from build123d import *

# Parameters (mm, degrees)
CROQUIS1_R                 = 8
SALIENTE_EXTRUIR1_DEPTH    = 20
CORTAR_EXTRUIR1_DEPTH      = 8.5
CROQUIS3_R                 = 6.75
CORTAR_EXTRUIR2_DEPTH      = 9
CORTAR_EXTRUIR3_REACH      = 17.78
CROQUIS4_R                 = 2.025
CORTAR_EXTRUIR4_DEPTH      = 9
CORTAR_EXTRUIR4_DEPTH_BACK = 23.978250586
CROQUIS5_R                 = 2
SALIENTE_EXTRUIR2_START    = 7
CROQUIS6_R                 = 8
CROQUIS6_R_2               = 6.75
SALIENTE_EXTRUIR2_DEPTH    = 7


with BuildPart() as part:
    # Croquis1 → Saliente-Extruir1 (new body)
    with BuildSketch(Plane(origin=(0, 0, 0), x_dir=(0, 0, -1), z_dir=(1, 0, 0))):
        Circle(CROQUIS1_R)
    extrude(amount=SALIENTE_EXTRUIR1_DEPTH)

    # Croquis2 → Cortar-Extruir1 (cut)
    with BuildSketch(Plane(origin=(20, 0, 0), x_dir=(0, 0, -1), z_dir=(1, 0, 0))):
        Polygon((0, -6.957070744), (6.025, -3.478535372), (6.025, 3.478535372), (0, 6.957070744), (-6.025, 3.478535372), (-6.025, -3.478535372), align=None)
    extrude(amount=-CORTAR_EXTRUIR1_DEPTH, mode=Mode.SUBTRACT)

    # Croquis3 → Cortar-Extruir2 (cut)
    with BuildSketch(Plane.ZY):
        Circle(CROQUIS3_R)
    extrude(amount=-CORTAR_EXTRUIR2_DEPTH, mode=Mode.SUBTRACT)

    # Croquis4 → Cortar-Extruir3 (cut, up to next)
    with BuildSketch(Plane.ZY.offset(-9), mode=Mode.PRIVATE) as cortar_extruir3_sk1:
        Circle(CROQUIS4_R)
    cortar_extruir3_tool1 = extrude(cortar_extruir3_sk1.sketch, amount=-CORTAR_EXTRUIR3_REACH, mode=Mode.PRIVATE) & part.part
    add(cortar_extruir3_tool1.solids().sort_by_distance((9, 0, 0))[0], mode=Mode.SUBTRACT)

    # Croquis5 → Cortar-Extruir4 (cut, two sides: drawn at the far end of the back side and taken through both)
    with BuildSketch(Plane.XY.offset(-CORTAR_EXTRUIR4_DEPTH_BACK)):
        with Locations(Location((2.1, 0, 0), (0, 0, 180))):
            Circle(CROQUIS5_R)
    extrude(amount=CORTAR_EXTRUIR4_DEPTH + CORTAR_EXTRUIR4_DEPTH_BACK, mode=Mode.SUBTRACT)

    # Croquis6 → Saliente-Extruir2 (add)
    with BuildSketch(Plane.ZY.offset(SALIENTE_EXTRUIR2_START)):
        Circle(CROQUIS6_R)
        Circle(CROQUIS6_R_2, mode=Mode.SUBTRACT)
    extrude(amount=-SALIENTE_EXTRUIR2_DEPTH)


solid = part.part
Input: part model. Units: mm. Frame: model coordinates. A direction names the side the tool comes from. Give positions to 0.01 mm unless a question says otherwise; leave off trailing zeros. Order: outer loops, then holes, each group sorted by start corner. A loop starts at its lowest first (then second) coordinate and runs counter-clockwise, first axis right, second up. Notation, with made-up numbers: (21, 52.25) - (72, 52.25) arc R26 ccw to (72, 75.25) - close; hole circle Ø7 at (-21, 27.25). An arc over 180 degrees is marked (long way). Answer as a JSON object with one key per item and string values. Group by question number.
Q1. Set-up query: faces 4 (the face through (9, 2, 1)), 5 (the face through (15.81, -5.193, 3.055)), 6 (the face through (0.253, 0.766, -7.234)). Return all of +Z, -Z, +X, -X, +Y, -Y with unobstructed straight access to the full face (end or side cutting, diameter ignored); none if empty.
Q2. Line query: probe 1 along Y at (x, z) = (2.1, -7.2); probe 2 along Y at (x, z) = (5.25, 0). Output: solid intervals per line, ascending.
Q3. Mould query, pull axis X, two halves, no side actions, for faces 1 (the face through (11.5, 2, 1)), 2 (the face through (15.81, 5.242, 2.97)), 3 (the face through (2.534, 1.952, 7.213)). Classes: pulls with the +X half, pulls with the -X half, needs draft (parallel to the pull), parting line crosses it, or undercut.
Q4. Cut plane A-A, the plane y = 0. Output: boundary loops of the cut face in (x, z) (3 decimals), then the cut area to 4 significant figures.
Q5. Cut plane B-B, the plane x = 14.75. Output: boundary loops of the cut face in (y, z) (3 decimals), then the cut area to 3 significant figures.
Q6. Cut plane D-D, the plane x = 2.1. Output: boundary loops of the cut face in (y, z), then the cut area to 3 significant figures.
Q7. Cut plane C-C, the plane z = 1.5. Output: boundary loops of the cut face in (x, y).
Q8. First-contact query: pin 1 Ø1 at (x, y) = (16.5, -3.5) entering from +Z; pin 2 Ø5 at (x, z) = (10.5, -4.5) entering from -Y; pin 3 Ø5 at (x, z) = (15, -3.5) entering from -Y. Flat tips, straight axial feed; report the tip coordinate or a pass-through.
Results:
{
 "1": {"face 4": "-X", "face 5": "+X", "face 6": "+Z, -Z"},
 "2": {"probe 1": "-3.49 to -2, 2 to 3.49", "probe 2": "-8 to -6.75, 6.75 to 8"},
 "3": {"face 1": "pulls with the +X half", "face 2": "needs draft", "face 3": "undercut"},
 "4": {"outline": "(-7, -8) - (0.1, -8) - (0.1, -6.75) - (-7, -6.75) - close; (-7, 6.75) - (0.1, 6.75) - (0.1, 8) - (-7, 8) - close; (4.1, -8) - (20, -8) - (20, -6.025) - (11.5, -6.025) - (11.5, -2.025) - (9, -2.025) - (9, -6.75) - (4.1, -6.75) - close; (4.1, 6.75) - (9, 6.75) - (9, 2.025) - (11.5, 2.025) - (11.5, 6.025) - (20, 6.025) - (20, 8) - (4.1, 8) - close", "area": "93.45 mm^2"},
 "5": {"outline": "circle Ø16 at (0, 0); hole (-6.957, 0) - (-3.479, -6.025) - (3.479, -6.025) - (6.957, 0) - (3.479, 6.025) - (-3.479, 6.025) - close", "area": "75.3 mm^2"},
 "6": {"outline": "(-2, -7.75) - (-2, -6.45) arc R6.75 cw to (-2, 6.45) - (-2, 7.75) arc R8 ccw to start; (2, -7.75) arc R8 ccw to (2, 7.75) - (2, 6.45) arc R6.75 cw to (2, -6.45) - close", "area": "47.8 mm^2"},
 "7": {"outline": "(-7, -7.86) - (20, -7.86) - (20, -6.09) - (11.5, -6.09) - (11.5, -1.36) - (9, -1.36) - (9, -6.58) - (-7, -6.58) - close; (-7, 6.58) - (9, 6.58) - (9, 1.36) - (11.5, 1.36) - (11.5, 6.09) - (20, 6.09) - (20, 7.86) - (-7, 7.86) - close"},
 "8": {"pin 1": "z = 7.42", "pin 2": "y = -7.75", "pin 3": "y = -7.94"}
}
